from build123d import *

# Parameters (mm, degrees)
ESQUISSE1_W               = 46.5
ESQUISSE1_H               = 28.6
BOSS_EXTRU_1_DEPTH        = 34
CHANFREIN1_SIZE           = 2
ESQUISSE2_R               = 10.5
BOSS_EXTRU_2_DEPTH        = 2
TROU_TARAUD_M2X0_41_D     = 1.6
TROU_TARAUD_M2X0_41_DEPTH = 3.2
TROU_TARAUD_M2X0_41_TIP   = 0.480688495


with BuildPart() as part:
    # Esquisse1 → Boss.-Extru.1 (new body)
    with BuildSketch(Plane(origin=(0, 0, 0), x_dir=(1, 0, 0), z_dir=(0, 1, 0))):
        Rectangle(ESQUISSE1_W, ESQUISSE1_H)
    extrude(amount=BOSS_EXTRU_1_DEPTH)

    # Chanfrein1
    chanfrein1_edges = [part.edges().sort_by_distance(p)[0] for p in [
        (23.25, 17, 14.3),
        (-23.25, 17, 14.3),
        (-23.25, 17, -14.3),
        (23.25, 17, -14.3),
    ]]
    chamfer(chanfrein1_edges, length=CHANFREIN1_SIZE)

    # Esquisse2 → Boss.-Extru.2 (add)
    with BuildSketch(Plane(origin=(0, 34, 0), x_dir=(1, 0, 0), z_dir=(0, 1, 0))):
        with Locations(Location((12.25, 0, 0), (0, 0, 90))):
            Circle(ESQUISSE2_R)
    extrude(amount=BOSS_EXTRU_2_DEPTH)

    # Trou taraudé M2x0.41
    with Locations(Plane(origin=(0, 36, 0), x_dir=(1, 0, 0), z_dir=(0, 1, 0))):
        with Locations((12.25, 8), (20.25, 0), (12.25, -8), (4.25, 0)):
            Hole(TROU_TARAUD_M2X0_41_D / 2, depth=TROU_TARAUD_M2X0_41_DEPTH)
            with Locations((0, 0, -(TROU_TARAUD_M2X0_41_DEPTH + TROU_TARAUD_M2X0_41_TIP / 2))):  # 118° drill point
                Cone(0, TROU_TARAUD_M2X0_41_D / 2, TROU_TARAUD_M2X0_41_TIP, mode=Mode.SUBTRACT)


solid = part.part
Can you work these out from the model? Positions are in its coordinate system, mm. A direction names the side the tool comes from. Coordinates: 2 decimals unless noted, no trailing zeros. Write each loop counter-clockwise with the first axis right and the second up, starting at its lowest first coordinate (ties: lowest second). Pieces come first, ordered by that corner, then holes. Notation, with made-up numbers: (87.25, 14.25) - (101.25, 14.25) arc R24 ccw to (101.25, 48.25) - close; hole circle Ø6 at (10, 10). An arc over 180 degrees is marked (long way). Return JSON: item names as keys, results as strings. Group by question number.
Item 1: If we section it at B-B (z = 2.5): Write out the boundary of the cut face in (x, y), then the cut area to 3 significant figures.
Item 2: If we section it at A-A (x = 14): Write out the boundary of the cut face in (y, z).
Item 3: If we section it at C-C (z = -11.75): Write out the boundary of the cut face in (x, y), then the cut area to 3 significant figures.
Item 4: Which directions (+Z, -Z, +X, -X, +Y, -Y) give clear straight access to the entire face, cutting with the end or side of a thin tool? Please do faces 4 (the face through (-22.24, 16.76, -13.31)), 5 (the face through (22.5, 34.99, 2.28)).
Item 5: We'd pull the mould along Z, two halves only. Please class faces 1 (the face through (23.25, 17, 0)), 2 (the face through (22.24, 16.76, -13.31)), 3 (the face through (12.354, 34.378, -8.793)): pulls with the +Z half, pulls with the -Z half, needs draft (parallel to the pull), parting line crosses it, or undercut.
Item 6: I'm going to push flat-ended pins straight in: pin 1 Ø8.5 at (x, z) = (-10, 1.5) entering from +Y; pin 2 Ø1.8 at (x, z) = (12.25, -8) entering from +Y; pin 3 Ø1 at (x, z) = (12.25, 8) entering from +Y; pin 4 Ø1.4 at (x, z) = (20.25, 0) entering from +Y. Where does each tip first touch, or does it pass through?
Item 7: Please list where these lines run through material, in increasing order: probe 1 along X at (y, z) = (33.8, -8); probe 2 along Z at (x, y) = (20.25, 33.75); probe 3 along Y at (x, z) = (-21, 1.75).
Item 8: If we section it at D-D (x = -11): Write out the boundary of the cut face in (y, z), then the cut area to 3 significant figures.
Return value:
{
 "1": {"outline": "(-23.25, 0) - (23.25, 0) - (23.25, 34) - (22.45, 34) - (22.45, 36) - (2.05, 36) - (2.05, 34) - (-23.25, 34) - close", "area": "1,620 mm^2"},
 "2": {"outline": "(0, -14.3) - (34, -14.3) - (34, -10.35) - (36, -10.35) - (36, 10.35) - (34, 10.35) - (34, 14.3) - (0, 14.3) - close"},
 "3": {"outline": "(-23.25, 0) - (23.25, 0) - (23.25, 34) - (-23.25, 34) - close", "area": "1,580 mm^2"},
 "4": {"face 4": "-Z, -X, +Y, -Y", "face 5": "+Y"},
 "5": {"face 1": "needs draft", "face 2": "pulls with the -Z half", "face 3": "undercut"},
 "6": {"pin 1": "stops at y = 34", "pin 2": "stops at y = 36", "pin 3": "stops at y = 32.62", "pin 4": "stops at y = 32.74"},
 "7": {"probe 1": "x = -23.25 to 11.45, 13.05 to 23.25", "probe 2": "z = -14.3 to -0.8, 0.8 to 14.3", "probe 3": "y = 0 to 34"},
 "8": {"outline": "(0, -14.3) - (34, -14.3) - (34, 14.3) - (0, 14.3) - close", "area": "972 mm^2"}
}
